Check sheet for the drawn part. Datum: minimum x, y, z corner. Units: mm. Give positions to 0.01 mm unless a question says otherwise; leave off trailing zeros. Write each loop counter-clockwise with the first axis right and the second up, starting at its lowest first coordinate (ties: lowest second). Pieces come first, ordered by that corner, then holes. Notation, with made-up numbers: M 65,78.25 L 82,78.25 A12 ccw 82,86.25 Z; hole C -11.5,-16 d7. An arc over 180 degrees is marked long. Write item = value, one per line. Start each with the question number.
1) Sectioned sample at A-A, the plane x = 62.5. Record the cut outline in (y, z).
2) Sectioned sample at B-B, the plane y = 62.5. Record the cut outline in (x, z).
3) Gauge pin test, flat end, axial feed: pin 1 (1 mm diameter, centred on x = 98.5, z = 0.5, fed in from +Y). Record the tip position at first contact, or that the pin passes through.
4) Scan lines: L1, parallel to Y at x = 62.5, z = 0.8; L2, parallel to X at y = 35, z = 0.6 (1 decimal); L3, parallel to X at y = 64, z = 0.45. Record each from-to range of solid material in increasing order.
5) Sectioned sample at D-D, the plane y = 35. Record the cut outline in (x, z) (1 decimal).
6) Sectioned sample at C-C, the plane x = 88. Record the cut outline in (y, z) (1 decimal), then the cut area to 3 significant figures.
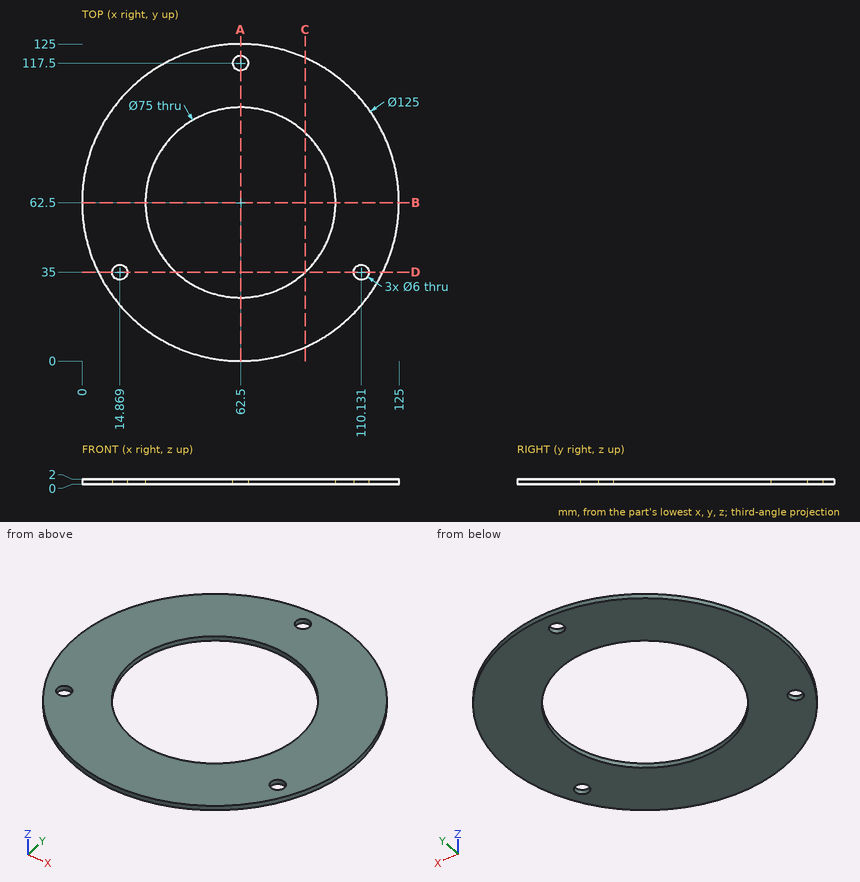
Data:
q1.outline = M 0,0 L 25,0 L 25,2 L 0,2 Z; M 100,0 L 114.5,0 L 114.5,2 L 100,2 Z; M 120.5,0 L 125,0 L 125,2 L 120.5,2 Z
q2.outline = M 0,0 L 25,0 L 25,2 L 0,2 Z; M 100,0 L 125,0 L 125,2 L 100,2 Z
q3.pin_1 = 113.94
q4.L1 = 0 to 25, 100 to 114.5, 120.5 to 125
q4.L2 = 6.4 to 11.9, 17.9 to 37, 88 to 107.1, 113.1 to 118.6
q4.L3 = 0.02 to 25.03, 99.97 to 124.98
q5.outline = M 6.4,0 L 11.9,0 L 11.9,2 L 6.4,2 Z; M 17.9,0 L 37,0 L 37,2 L 17.9,2 Z; M 88,0 L 107.1,0 L 107.1,2 L 88,2 Z; M 113.1,0 L 118.6,0 L 118.6,2 L 113.1,2 Z
q6.outline = M 5.4,0 L 35,0 L 35,2 L 5.4,2 Z; M 90,0 L 119.6,0 L 119.6,2 L 90,2 Z
q6.area = 118 mm2
